```python
from build123d import *

# Parameters (mm, degrees)
BOSS_EXTRUDE1_DEPTH = 6
BOSS_EXTRUDE2_START = 0.3
BOSS_EXTRUDE2_DEPTH = 1.6
SKETCH1_3_W         = 5
SKETCH1_3_H         = 1
BOSS_EXTRUDE3_DEPTH = 0.3
BOSS_EXTRUDE4_START = 1.9
SKETCH1_5_W         = 5
SKETCH1_5_H         = 1
BOSS_EXTRUDE4_DEPTH = 0.3
BOSS_EXTRUDE5_START = 2.2
BOSS_EXTRUDE5_DEPTH = 1.6
BOSS_EXTRUDE6_START = 3.8
SKETCH1_6_W         = 5
SKETCH1_6_H         = 1
BOSS_EXTRUDE6_DEPTH = 0.3
BOSS_EXTRUDE7_START = 4.1
BOSS_EXTRUDE7_DEPTH = 1.6
BOSS_EXTRUDE8_START = 5.7
SKETCH1_7_W         = 5
SKETCH1_7_H         = 1
BOSS_EXTRUDE8_DEPTH = 0.3
SKETCH3_W           = 2.4
SKETCH3_H           = 6
BOSS_EXTRUDE9_DEPTH = 0.2


with BuildPart() as part:
    # Sketch1 → Boss-Extrude1 (new body)
    with BuildSketch(Plane.XY):
        Polygon((5.5, 0.5), (0.5, 0.5), (0.5, 1.5), (0.5, 2), (0, 2), (0, 0), (6, 0), (6, 0.5), align=None)
    extrude(amount=BOSS_EXTRUDE1_DEPTH)

    # Sketch2 → Boss-Extrude2 (add)
    with BuildSketch(Plane.XY.offset(BOSS_EXTRUDE2_START)):
        with BuildLine():
            Line((5.833702875, 1.503863094), (6, 1.614972348))
            Line((6, 1.614972348), (5.082039937, 2.988882388))
            ThreePointArc((5.082039937, 2.988882388), (4.454237941, 3.298502565), (3.872198004, 2.909620177))
            Line((3.872198004, 2.909620177), (3.413156013, 1.97884273))
            ThreePointArc((3.413156013, 1.97884273), (3.228753823, 1.775395104), (2.964726016, 1.7))
            Line((2.964726016, 1.7), (1.4, 1.7))
            ThreePointArc((1.4, 1.7), (0.905025253, 1.494974747), (0.7, 1))
            Line((0.7, 1), (0.7, 0.5))
            Line((0.7, 0.5), (0.9, 0.5))
            Line((0.9, 0.5), (0.9, 1))
            ThreePointArc((0.9, 1), (1.046446609, 1.353553391), (1.4, 1.5))
            Line((1.4, 1.5), (2.964726016, 1.5))
            ThreePointArc((2.964726016, 1.5), (3.334364945, 1.605553146), (3.592528012, 1.890379823))
            Line((3.592528012, 1.890379823), (4.051570003, 2.82115727))
            ThreePointArc((4.051570003, 2.82115727), (4.467312815, 3.098930404), (4.915742812, 2.877773134))
            Line((4.915742812, 2.877773134), (5.833702875, 1.503863094))
        make_face()
    extrude(amount=BOSS_EXTRUDE2_DEPTH)

    # Sketch1<3> → Boss-Extrude3 (add)
    with BuildSketch(Plane.XY):
        with Locations((3, 1)):
            Rectangle(SKETCH1_3_W, SKETCH1_3_H)
        Polygon((0.5, 2), (0.5, 1.5), (5.5, 1.5), (5.5, 0.5), (6, 0.5), (6, 2), align=None)
    extrude(amount=BOSS_EXTRUDE3_DEPTH)

    # Sketch1<5> → Boss-Extrude4 (add)
    with BuildSketch(Plane.XY.offset(BOSS_EXTRUDE4_START)):
        Polygon((0.5, 2), (0.5, 1.5), (5.5, 1.5), (5.5, 0.5), (6, 0.5), (6, 2), align=None)
        with Locations((3, 1)):
            Rectangle(SKETCH1_5_W, SKETCH1_5_H)
    extrude(amount=BOSS_EXTRUDE4_DEPTH)

    # Sketch2<3> → Boss-Extrude5 (add)
    with BuildSketch(Plane.XY.offset(BOSS_EXTRUDE5_START)):
        with BuildLine():
            Line((5.833702875, 1.503863094), (6, 1.614972348))
            Line((6, 1.614972348), (5.082039937, 2.988882388))
            ThreePointArc((5.082039937, 2.988882388), (4.454237941, 3.298502565), (3.872198004, 2.909620177))
            Line((3.872198004, 2.909620177), (3.413156013, 1.97884273))
            ThreePointArc((3.413156013, 1.97884273), (3.228753823, 1.775395104), (2.964726016, 1.7))
            Line((2.964726016, 1.7), (1.4, 1.7))
            ThreePointArc((1.4, 1.7), (0.905025253, 1.494974747), (0.7, 1))
            Line((0.7, 1), (0.7, 0.5))
            Line((0.7, 0.5), (0.9, 0.5))
            Line((0.9, 0.5), (0.9, 1))
            ThreePointArc((0.9, 1), (1.046446609, 1.353553391), (1.4, 1.5))
            Line((1.4, 1.5), (2.964726016, 1.5))
            ThreePointArc((2.964726016, 1.5), (3.334364945, 1.605553146), (3.592528012, 1.890379823))
            Line((3.592528012, 1.890379823), (4.051570003, 2.82115727))
            ThreePointArc((4.051570003, 2.82115727), (4.467312815, 3.098930404), (4.915742812, 2.877773134))
            Line((4.915742812, 2.877773134), (5.833702875, 1.503863094))
        make_face()
    extrude(amount=BOSS_EXTRUDE5_DEPTH)

    # Sketch1<6> → Boss-Extrude6 (add)
    with BuildSketch(Plane.XY.offset(BOSS_EXTRUDE6_START)):
        with Locations((3, 1)):
            Rectangle(SKETCH1_6_W, SKETCH1_6_H)
        Polygon((0.5, 2), (0.5, 1.5), (5.5, 1.5), (5.5, 0.5), (6, 0.5), (6, 2), align=None)
    extrude(amount=BOSS_EXTRUDE6_DEPTH)

    # Sketch2<4> → Boss-Extrude7 (add)
    with BuildSketch(Plane.XY.offset(BOSS_EXTRUDE7_START)):
        with BuildLine():
            Line((5.833702875, 1.503863094), (6, 1.614972348))
            Line((6, 1.614972348), (5.082039937, 2.988882388))
            ThreePointArc((5.082039937, 2.988882388), (4.454237941, 3.298502565), (3.872198004, 2.909620177))
            Line((3.872198004, 2.909620177), (3.413156013, 1.97884273))
            ThreePointArc((3.413156013, 1.97884273), (3.228753823, 1.775395104), (2.964726016, 1.7))
            Line((2.964726016, 1.7), (1.4, 1.7))
            ThreePointArc((1.4, 1.7), (0.905025253, 1.494974747), (0.7, 1))
            Line((0.7, 1), (0.7, 0.5))
            Line((0.7, 0.5), (0.9, 0.5))
            Line((0.9, 0.5), (0.9, 1))
            ThreePointArc((0.9, 1), (1.046446609, 1.353553391), (1.4, 1.5))
            Line((1.4, 1.5), (2.964726016, 1.5))
            ThreePointArc((2.964726016, 1.5), (3.334364945, 1.605553146), (3.592528012, 1.890379823))
            Line((3.592528012, 1.890379823), (4.051570003, 2.82115727))
            ThreePointArc((4.051570003, 2.82115727), (4.467312815, 3.098930404), (4.915742812, 2.877773134))
            Line((4.915742812, 2.877773134), (5.833702875, 1.503863094))
        make_face()
    extrude(amount=BOSS_EXTRUDE7_DEPTH)

    # Sketch1<7> → Boss-Extrude8 (add)
    with BuildSketch(Plane.XY.offset(BOSS_EXTRUDE8_START)):
        Polygon((0.5, 2), (0.5, 1.5), (5.5, 1.5), (5.5, 0.5), (6, 0.5), (6, 2), align=None)
        with Locations((3, 1)):
            Rectangle(SKETCH1_7_W, SKETCH1_7_H)
    extrude(amount=BOSS_EXTRUDE8_DEPTH)

    # Sketch3 → Boss-Extrude9 (add)
    with BuildSketch(Plane(origin=(0, 2, 0), x_dir=(1, 0, 0), z_dir=(0, 1, 0))):
        with Locations((1.2, -3)):
            Rectangle(SKETCH3_W, SKETCH3_H)
    extrude(amount=-BOSS_EXTRUDE9_DEPTH)


solid = part.part
```
Input: part model. Units: mm. Frame: model coordinates. A direction names the side the tool comes from. Coordinates: 2 decimals unless noted, no trailing zeros. Loops run counter-clockwise (first coordinate to the right, second up) from the corner with the lowest first, then second, coordinate; pieces in that order, holes last.
Q1. Set-up query: faces 1 (the flat face through (5.37, 2.2, 2.99)), 2 (the cylindrical face through (4.5, 3.1, 1.1)), 3 (the flat face through (3, 0.5, 1)). Return all of +Z, -Z, +X, -X, +Y, -Y with unobstructed straight access to the full face (end or side cutting, diameter ignored); none if empty.
Results are:
face 1: none
face 2: +Z, -Z
face 3: +X
Q2. Section B-B, the plane y = 0.85. Return the cut outline in (x, z).
Results are:
outline: (0, 0) - (6, 0) - (6, 0.3) - (0.9, 0.3) - (0.9, 1.9) - (6, 1.9) - (6, 2.2) - (0.9, 2.2) - (0.9, 3.8) - (6, 3.8) - (6, 4.1) - (0.9, 4.1) - (0.9, 5.7) - (6, 5.7) - (6, 6) - (0, 6) - close; hole (0.5, 0.3) - (0.7, 0.3) - (0.7, 1.9) - (0.5, 1.9) - close; hole (0.5, 2.2) - (0.7, 2.2) - (0.7, 3.8) - (0.5, 3.8) - close; hole (0.5, 4.1) - (0.7, 4.1) - (0.7, 5.7) - (0.5, 5.7) - close
Q3. Line query: line 1 along Z through (x, y) = (1.05, 1.65); line 2 along X through (y, z) = (0.7, 3.45); line 3 along X through (y, z) = (1.85, 3.3). Output: solid intervals per line, ascending.
Results are:
line 1: z = 0 to 0.3, 1.9 to 2.2, 3.8 to 4.1, 5.7 to 6
line 2: x = 0 to 0.5, 0.7 to 0.9
line 3: x = 0 to 2.4, 3.32 to 3.57, 5.6 to 5.84
Q4. Contact query for flat-ended pins moving along their axis: pin 1 (1 mm diameter, centred on x = 4, y = 3, fed in from +Z); pin 2 (1.8 mm diameter, centred on x = 2, z = 2, fed in from +Y); pin 3 (1.4 mm diameter, centred on x = 4.5, y = 3, fed in from -Z). Output: stop coordinate, or through.
Results are:
pin 1: stops at z = 5.7
pin 2: stops at y = 2
pin 3: stops at z = 0.3
Q5. Section D-D, the plane x = 5. Return the cut outline in (y, z), and give its area (3 significant figures).
Results are:
outline: (0, 0) - (2, 0) - (2, 0.3) - (0.5, 0.3) - (0.5, 1.9) - (2, 1.9) - (2, 2.2) - (0.5, 2.2) - (0.5, 3.8) - (2, 3.8) - (2, 4.1) - (0.5, 4.1) - (0.5, 5.7) - (2, 5.7) - (2, 6) - (0, 6) - close; (2.75, 0.3) - (3.09, 0.3) - (3.09, 1.9) - (2.75, 1.9) - close; (2.75, 2.2) - (3.09, 2.2) - (3.09, 3.8) - (2.75, 3.8) - close; (2.75, 4.1) - (3.09, 4.1) - (3.09, 5.7) - (2.75, 5.7) - close
area: 6.42 mm2
Q6. Section A-A, the plane x = 2. Return the cut outline in (y, z).
Results are:
outline: (0, 0) - (2, 0) - (2, 6) - (0, 6) - close; hole (0.5, 0.3) - (1.5, 0.3) - (1.5, 1.9) - (0.5, 1.9) - close; hole (0.5, 2.2) - (1.5, 2.2) - (1.5, 3.8) - (0.5, 3.8) - close; hole (0.5, 4.1) - (1.5, 4.1) - (1.5, 5.7) - (0.5, 5.7) - close; hole (1.7, 0.3) - (1.8, 0.3) - (1.8, 1.9) - (1.7, 1.9) - close; hole (1.7, 2.2) - (1.8, 2.2) - (1.8, 3.8) - (1.7, 3.8) - close; hole (1.7, 4.1) - (1.8, 4.1) - (1.8, 5.7) - (1.7, 5.7) - close
Q7. Section C-C, the plane z = 1.7. Return the cut outline in (x, y).
Results are:
outline: (0, 0) - (6, 0) - (6, 0.5) - (0.9, 0.5) - (0.9, 1) arc R0.5 cw to (1.4, 1.5) - (2.96, 1.5) arc R0.7 ccw to (3.59, 1.89) - (4.05, 2.82) arc R0.5 cw to (4.92, 2.88) - (5.83, 1.5) - (6, 1.61) - (5.08, 2.99) arc R0.7 ccw to (3.87, 2.91) - (3.41, 1.98) arc R0.5 cw to (2.96, 1.7) - (1.4, 1.7) arc R0.7 ccw to (0.7, 1) - (0.7, 0.5) - (0.5, 0.5) - (0.5, 1.8) - (2.4, 1.8) - (2.4, 2) - (0, 2) - close
Q8. Mould query, pull axis X, two halves, no side actions, for faces 4 (the flat face through (2, 1.5, 3)), 5 (the flat face through (0.5, 1, 3)), 6 (the cylindrical face through (4.5, 3.3, 1.1)). Classes: +X half, -X half, draft (parallel to the pull), parting line (faces both ways), or undercut.
Results are:
face 4: draft
face 5: undercut
face 6: parting line
